```python
from build123d import *

# Parameters (mm, degrees)
SKETCH1_R           = 7.5
SKETCH1_R_2         = 5
SKETCH1_R_3         = 1.5
BOSS_EXTRUDE1_DEPTH = 6.1
SKETCH2_R           = 5.25
BOSS_EXTRUDE2_DEPTH = 2.5
BOSS_EXTRUDE3_DEPTH = 2.85
SKETCH3_R           = 4
SKETCH3_R_2         = 2.425
SKETCH3_R_3         = 0.875
CUT_EXTRUDE1_DEPTH  = 8
FILLET1_R           = 4
SKETCH5_R           = 3
BOSS_EXTRUDE4_DEPTH = 3


with BuildPart() as part:
    # Sketch1 → Boss-Extrude1 (new body)
    with BuildSketch(Plane(origin=(0, 0, 0), x_dir=(1, 0, 0), z_dir=(0, 1, 0))):
        Circle(SKETCH1_R)
        with Locations((-10.5, 0)):
            Circle(SKETCH1_R_2)
        with Locations((-10.5, 0)):
            Circle(SKETCH1_R_3, mode=Mode.SUBTRACT)
        with Locations((10.5, 0)):
            Circle(SKETCH1_R_2)
        with Locations((10.5, 0)):
            Circle(SKETCH1_R_3, mode=Mode.SUBTRACT)
    extrude(amount=BOSS_EXTRUDE1_DEPTH)

    # Sketch2 → Boss-Extrude2 (add)
    with BuildSketch(Plane(origin=(0, 6.1, 0), x_dir=(1, 0, 0), z_dir=(0, 1, 0))):
        Circle(SKETCH2_R)
    extrude(amount=BOSS_EXTRUDE2_DEPTH)

    # Sketch4 → Boss-Extrude3 (add)
    with BuildSketch(Plane.XZ):
        with BuildLine():
            Line((-2.291287847, -5), (2.291287847, -5))
            ThreePointArc((2.291287847, -5), (4.628827236, -2.970514841), (5.5, 0))
            ThreePointArc((5.5, 0), (4.628827236, 2.970514841), (2.291287847, 5))
            Line((2.291287847, 5), (-2.291287847, 5))
            ThreePointArc((-2.291287847, 5), (-4.628827236, 2.970514841), (-5.5, 0))
            ThreePointArc((-5.5, 0), (-4.628827236, -2.970514841), (-2.291287847, -5))
        make_face()
    extrude(amount=BOSS_EXTRUDE3_DEPTH)

    # Sketch3 → Cut-Extrude1 (cut)
    with BuildSketch(Plane(origin=(0, 8.6, 0), x_dir=(1, 0, 0), z_dir=(0, 1, 0))):
        Circle(SKETCH3_R)
        Circle(SKETCH3_R_2, mode=Mode.SUBTRACT)
        Circle(SKETCH3_R_3)
    extrude(amount=-CUT_EXTRUDE1_DEPTH, mode=Mode.SUBTRACT)

    # Fillet1
    fillet1_edges = [part.edges().sort_by_distance(p)[0] for p in [
        (-6.738095238, 3.05, -3.293641232),
        (6.738095238, 3.05, -3.293641232),
        (6.738095238, 3.05, 3.293641232),
        (-6.738095238, 3.05, 3.293641232),
    ]]
    fillet(fillet1_edges, radius=FILLET1_R)

    # Sketch5 → Boss-Extrude4 (add)
    with BuildSketch(Plane.XZ.offset(2.85)):
        Circle(SKETCH5_R)
        with BuildLine():
            ThreePointArc((0, -3), (-3, 0), (0, 3))
            Line((0, 3), (-4.609772229, 3))
            ThreePointArc((-4.609772229, 3), (-5.5, 0), (-4.609772229, -3))
            Line((-4.609772229, -3), (0, -3))
        make_face()
    extrude(amount=BOSS_EXTRUDE4_DEPTH)


solid = part.part
```
Design review of the part built by this model. Coordinates are the model's own, in mm. A direction names the side the tool comes from. Round coordinates to 2 decimals unless told otherwise and drop trailing zeros. Write each loop counter-clockwise with the first axis right and the second up, starting at its lowest first coordinate (ties: lowest second). Pieces come first, ordered by that corner, then holes.
Item 1: For faces 4 (the flat face through (0, -1, -5)), 5 (the cylindrical face through (0.1, 3, -7.5)), 6 (the cylindrical face through (3, -4, 0)), 7 (the flat face through (2, 0.6, 2)), 8 (the flat face through (0, -1, 5)), list the 3-axis set-ups (+Z, -Z, +X, -X, +Y, -Y) from which the entire face can be reached by the end or side of a thin tool; tool diameter is ignored.
Item 2: We need section C-C on y = 1.5. State how many separate pieces and enclosed holes the cut face has, and give its area (3 significant figures).
Item 3: We need section D-D on z = 6. Write out the cut boundary in (x, y), and give its area (3 significant figures).
Item 4: For probe 1 along Z at (x, y) = (0, 6) (3 decimals); probe 2 along Z at (x, y) = (-10.5, 2.25); probe 3 along X at (y, z) = (0.5, -0.75), list the stretches that pass through material, from the lowest coordinate up.
Item 5: Clearance check with flat-ended pins moving along their axes: pin 1 Ø3 at (y, z) = (-3.5, -3.5) entering from +X; pin 2 Ø0.9 at (x, y) = (-1.5, -4) entering from +Z; pin 3 Ø1.5 at (x, z) = (12, 5) entering from -Y. State where each tip first meets the part, or that it passes through.
Item 6: We need section A-A on x = 10.5. Write out the cut boundary in (y, z).
Item 7: We need section B-B on y = 7.25. Write out the cut boundary in (x, z) (3 decimals).
Item 8: The part is to be moulded in two halves that separate along Z. For faces 1 (the cylindrical face through (-12, 3, 0)), 2 (the flat face through (-2, -4, -3)), 3 (the flat face through (4, -2.85, 0)), say which applies: +Z half, -Z half, draft (parallel to the pull), parting line (faces both ways), or undercut.
Returned:
1. face 4: -Z, +X, -X, -Y
1. face 5: -Z, +Y, -Y
1. face 6: +X, -Y
1. face 7: +Y
1. face 8: +Z, +X, -X, -Y
2. separate pieces: 2
2. enclosed holes: 4
2. area: 274 mm2
3. outline: (-4.5, 0) - (4.5, 0) - (4.5, 6.1) - (-4.5, 6.1) - close
3. area: 54.9 mm2
4. probe 1: z = -7.5 to -4, -2.425 to -0.875, 0.875 to 2.425, 4 to 7.5
4. probe 2: z = -5 to -1.5, 1.5 to 5
4. probe 3: x = -15.44 to -11.8, -9.2 to 9.2, 11.8 to 15.44
5. pin 1: stops at x = 5.06
5. pin 2: stops at z = 3
5. pin 3: stops at y = 0
6. outline: (0, -5) - (6.1, -5) - (6.1, -1.5) - (0, -1.5) - close; (0, 1.5) - (6.1, 1.5) - (6.1, 5) - (0, 5) - close
7. outline: circle Ø10.5 at (0, 0); circle Ø4.85 at (0, 0); hole circle Ø8 at (0, 0); hole circle Ø1.75 at (0, 0)
8. face 1: undercut
8. face 2: -Z half
8. face 3: draft
